Verification items for the finished model (mm, model axes). Face numbers are marked on the shaded views. Coordinates: 2 decimals unless noted, no trailing zeros. Order: outer loops, then holes, each group sorted by start corner. A loop starts at its lowest first (then second) coordinate and runs counter-clockwise, first axis right, second up. Notation, with made-up numbers: M 55,86 L 62,86 A19 ccw 62,90 Z; hole C 81,-28 d4. An arc over 180 degrees is marked long. Return JSON: item names as keys, results as strings.
Autodesk Fusion 360 part; units mm, degrees
sketch "Sketch1" plane through (0, 0, 0) normal (0, 0, 1) x (1, 0, 0)
  line L0 (0.2, 0) -> (16.4, 0)
  line L1 (16.6, 0.2) -> (16.6, 16.4)
  line L2 (16.4, 16.6) -> (0.2, 16.6)
  line L3 (0, 16.4) -> (0, 0.2)
  arc A0 (0.2, 16.6) -> (0, 16.4) centre (0.2, 16.4) ccw
  arc A1 (16.6, 16.4) -> (16.4, 16.6) centre (16.4, 16.4) ccw
  arc A2 (16.4, 0) -> (16.6, 0.2) centre (16.4, 0.2) ccw
  arc A3 (0, 0.2) -> (0.2, 0) centre (0.2, 0.2) ccw
  line L4 (16.4, 17.25) -> (0.2, 17.25)
  arc A4 (0.2, 17.25) -> (-0.65, 16.4) centre (0.2, 16.4) ccw
  line L5 (-0.65, 16.4) -> (-0.65, 0.2)
  arc A5 (-0.65, 0.2) -> (0.2, -0.65) centre (0.2, 0.2) ccw
  line L6 (0.2, -0.65) -> (16.4, -0.65)
  arc A6 (16.4, -0.65) -> (17.25, 0.2) centre (16.4, 0.2) ccw
  line L7 (17.25, 0.2) -> (17.25, 16.4)
  arc A7 (17.25, 16.4) -> (16.4, 17.25) centre (16.4, 16.4) ccw
  line L8 (14.4, 14.4) -> (2.2, 14.4)
  line L9 (2.2, 14.4) -> (2.2, 2.2)
  line L10 (2.2, 2.2) -> (14.4, 2.2)
  line L11 (14.4, 2.2) -> (14.4, 14.4)
  line L12 (0.2, -5) -> (16.4, -5)
  arc A8 (16.4, -5) -> (21.6, 0.2) centre (16.4, 0.2) ccw
  line L13 (21.6, 0.2) -> (21.6, 16.4)
  arc A9 (21.6, 16.4) -> (16.4, 21.6) centre (16.4, 16.4) ccw
  line L14 (16.4, 21.6) -> (0.2, 21.6)
  arc A10 (0.2, 21.6) -> (-5, 16.4) centre (0.2, 16.4) ccw
  line L15 (-5, 16.4) -> (-5, 0.2)
  arc A11 (-5, 0.2) -> (0.2, -5) centre (0.2, 0.2) ccw
  point P0 (16.6, 0)
  point P1 (0, 16.6)
  dimension "d1" = 16.6
  dimension "d2" = 16.6
  dimension "d3" = 0.2
  dimension "d4" = 0.65
  dimension "d5" = -2.2
  dimension "d15" = 5
extrude "Extrude1" add sketch "Sketch1" along normal blind 0.35 contours L0 L1 L2 L3 A0 A1 A2 A3 | L4 A4 L5 A5 L6 A6 L7 A7
extrude "Extrude2" add sketch "Sketch1" against normal blind 1.35 contours L4 A4 L5 A5 L6 A6 L7 A7
fillet "Fillet1" radius 2 4 edges at (2.2, 14.4, 0.175) (14.4, 14.4, 0.175) (14.4, 2.2, 0.175) (2.2, 2.2, 0.175)
chamfer "Chamfer1" distance 0.35 angle 45 8 edges at (8.3, 14.4, 0.35) (13.8142, 13.8142, 0.35) (14.4, 8.3, 0.35) (13.8142, 2.7858, 0.35) (8.3, 2.2, 0.35) (2.7858, 2.7858, 0.35) (2.2, 8.3, 0.35) (2.7858, 13.8142, 0.35)
extrude "Extrude3" add 1 faces at (17.0333, 5.6, -1.35) along direction (0, 0, -1) blind 0.3 draft 30
extrude "Extrude4" cut sketch "Sketch1" against normal blind 6 contours L12 A8 L13 A9 L14 A10 L15 A11
chamfer "Chamfer2" distance 0.1 angle 45 8 edges at (8.3, 16.4268, -1.65) (0.1811, 16.4189, -1.65) (0.1732, 8.3, -1.65) (0.1811, 0.1811, -1.65) (8.3, 0.1732, -1.65) (16.4189, 0.1811, -1.65) (16.4268, 8.3, -1.65) (16.4189, 16.4189, -1.65)
sketch "Sketch2" plane through (0, 0, -1.65) normal (0, 0, -1) x (1, 0, 0)
  line L0 (17.25, -16.4) -> (17.25, -0.2)
  arc A0 (17.25, -0.2) -> (16.4, 0.65) centre (16.4, -0.2) ccw
  line L1 (16.4, 0.65) -> (0.2, 0.65)
  arc A1 (0.2, 0.65) -> (-0.65, -0.2) centre (0.2, -0.2) ccw
  line L2 (-0.65, -0.2) -> (-0.65, -16.4)
  arc A2 (-0.65, -16.4) -> (0.2, -17.25) centre (0.2, -16.4) ccw
  line L3 (0.2, -17.25) -> (16.4, -17.25)
  arc A3 (16.4, -17.25) -> (17.25, -16.4) centre (16.4, -16.4) ccw
  line L4 (16.4, -16.5268) -> (0.2, -16.5268)
  arc A4 (0.0732, -16.4) -> (0.2, -16.5268) centre (0.2, -16.4) ccw
  line L5 (0.0732, -16.4) -> (0.0732, -0.2)
  arc A5 (0.2, -0.0732) -> (0.0732, -0.2) centre (0.2, -0.2) ccw
  line L6 (0.2, -0.0732) -> (16.4, -0.0732)
  arc A6 (16.5268, -0.2) -> (16.4, -0.0732) centre (16.4, -0.2) ccw
  line L7 (16.5268, -0.2) -> (16.5268, -16.4)
  arc A7 (16.4, -16.5268) -> (16.5268, -16.4) centre (16.4, -16.4) ccw
  line L8 (8.3, 0.65) -> (8.3, -17.25) construction
  line L9 (7.7, -17.25) -> (7.7, 0.65)
  line L10 (8.9, -17.25) -> (8.9, 0.65)
  line L11 (8.3, -8.3) -> (0.2, 0.65)
  line L12 (8.3, -8.3) -> (-0.65, -0.2)
  line L13 (8.3, -8.3) -> (-0.65, -16.4)
  line L14 (8.3, -8.3) -> (0.2, -17.25)
  line L15 (8.3, -8.3) -> (16.4, -17.25)
  line L16 (8.3, -8.3) -> (17.25, -16.4)
  line L17 (8.3, -8.3) -> (17.25, -0.2)
  line L18 (8.3, -8.3) -> (16.4, 0.65)
  point P0 (0.5, -16.2)
  point P1 (0.5, -0.5)
  point P2 (16.2, -0.5)
  point P3 (16.2, -16.2)
  dimension "d19" = 0.6
  dimension "d23" = 360
extrude "Extrude5" cut sketch "Sketch2" against normal up to surface (1.65 mm away) contours L3 L4 L9 L10 | L1 L6 L9 L10 | L4 L9 L10 L14 L15 | L6 L9 L10 L11 L18
equation "d1 = d2"
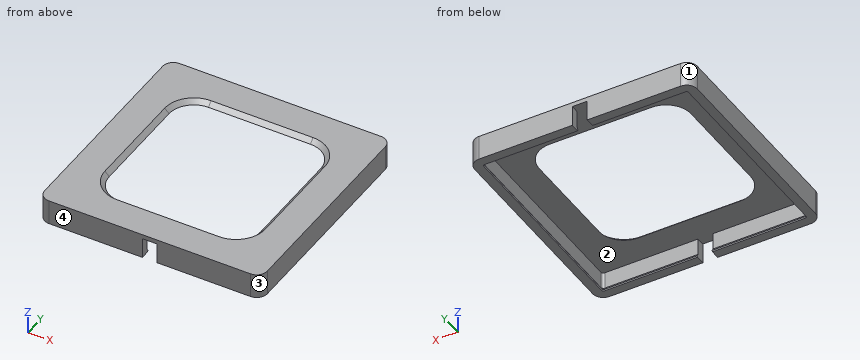
Q1. Cross-section at B-B, the plane z = -1.1. Record the boundary of the cut face in (x, y).
Values:
{"outline": "M -0.65,0.2 A0.85 ccw 0.2,-0.65 L 7.7,-0.65 L 7.7,0 L 0.2,0 A0.2 cw 0,0.2 L 0,16.4 A0.2 cw 0.2,16.6 L 7.7,16.6 L 7.7,17.25 L 0.2,17.25 A0.85 ccw -0.65,16.4 Z; M 8.9,-0.65 L 16.4,-0.65 A0.85 ccw 17.25,0.2 L 17.25,16.4 A0.85 ccw 16.4,17.25 L 8.9,17.25 L 8.9,16.6 L 16.4,16.6 A0.2 cw 16.6,16.4 L 16.6,0.2 A0.2 cw 16.4,0 L 8.9,0 Z"}
Q2. Cross-section at D-D, the plane x = 1. Record the boundary of the cut face in (y, z).
Values:
{"outline": "M -0.65,-1.65 L 0.07,-1.65 L 0.12,-1.56 L 0,-1.35 L 0,0 L 16.6,0 L 16.6,-1.35 L 16.48,-1.56 L 16.53,-1.65 L 17.25,-1.65 L 17.25,0.35 L -0.65,0.35 Z"}
Q3. Draft check along X on the marked faces 1, 2, 3 and 4. Enter one of: pulls with the +X half, pulls with the -X half, needs draft (parallel to the pull), parting line crosses it, or undercut.
Values:
{"face 1": "pulls with the -X half", "face 2": "undercut", "face 3": "pulls with the +X half", "face 4": "needs draft"}
Q4. Go/stop test with a flat-tipped pin: pin 1 (5 mm diameter, centred on x = 4.5, y = 12, fed in from -Z). Record where the tip stops, or that it passes through.
Values:
{"pin 1": "z = 0"}
Q5. Material ranges on line 1 along Y through (x, z) = (4.25, -0.2); line 2 along Z through (x, y) = (11.5, 1.25), recorded low to high.
Values:
{"line 1": "-0.65 to 0, 16.6 to 17.25", "line 2": "0 to 0.35"}
